Here's how the part is built. I have some questions about the finished solid (model axes, mm). Face numbers are marked on the shaded views. A direction names the side the tool comes from. Coordinates: 2 decimals unless noted, no trailing zeros. Loops run counter-clockwise (first coordinate to the right, second up) from the corner with the lowest first, then second, coordinate; pieces in that order, holes last. Notation, with made-up numbers: M 49,53.25 L 62,53.25 A33 cw 62,86.25 Z; hole C 76.25,-1 d3. An arc over 180 degrees is marked long. Use CSV: the item, a comma, the result in double quotes. Start each with the question number.
Q1. If we section it at C-C (z = -30): Please give me the cut outline in (x, y), and give its area (3 significant figures).
Q2. If we section it at A-A (x = 15): Please give me the cut outline in (y, z), and give its area (3 significant figures).
Q3. For pin 1 Ø2.5 at (x, z) = (9, -43.5) entering from -Y; pin 2 Ø1.5 at (x, z) = (11, -41.5) entering from +Y; pin 3 Ø8 at (x, y) = (7.5, 5) entering from -Z, each with a flat end and sliding along its axis, tell me the tip position at first contact or that it passes through.
Q4. Which directions (+Z, -Z, +X, -X, +Y, -Y) give clear straight access to the entire face, cutting with the end or side of a thin tool? Please do the marked faces 1, 2, 3 and 4.
Q5. If we section it at D-D (x = 10): Please give me the cut outline in (y, z), and give its area (3 significant figures).
Q6. Please list where these lines run through material, in increasing order: probe 1 along X at (y, z) = (28.55, 4.75); probe 2 along X at (y, z) = (28, 4); probe 3 along Z at (x, y) = (5.25, 11.5). Write a range as [from, to].
Q7. If we section it at B-B (y = 22): Please give me the cut outline in (x, z), and give its area (3 significant figures).
Q8. If we mould it in two halves opening along Y, with no side actions, what happens to the marked faces 5, 6 and 7? For each: +Y half, -Y half, draft (parallel to the pull), parting line (faces both ways), or undercut.
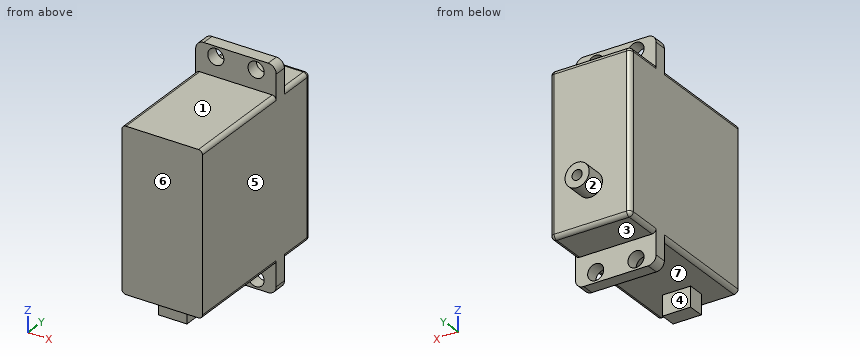
Autodesk Inventor part; units mm, degrees
ref_plane "作業平面1" through (0, 27.8, 0) normal (0, -1, 0) x (1, 0, 0)
ref_plane "作業平面2" through (0, 40.5, -20) normal (0, 0, 1) x (1, 0, 0)
ref_plane "作業平面3" through (0, 8, 0) normal (0, -1, 0) x (1, 0, 0)
sketch "スケッチ1" plane through (0, 0, 0) normal (0, 1, 0) x (-1, 0, 0)
  line L0 (0, 0) -> (-20, 0)
  line L1 (-20, 0) -> (-20, -40)
  line L2 (-20, -40) -> (0, -40)
  line L3 (0, -40) -> (0, 0)
  line L4 (0, -44.75) -> (-20, -44.75)
  line L5 (-20, -44.75) -> (-20, 4.75)
  line L6 (-20, 4.75) -> (0, 4.75)
  line L7 (0, 4.75) -> (0, -44.75)
  line L8 (-2, -47.25) -> (-18, -47.25)
  line L9 (-20, -45.25) -> (-20, 5.25)
  line L10 (-18, 7.25) -> (-2, 7.25)
  line L11 (0, 5.25) -> (0, -45.25)
  line L12 (-10, -61.4419) -> (-10, 22.3426)
  arc A0 (0, 5.25) -> (-2, 7.25) centre (-2, 5.25) ccw
  arc A1 (-18, 7.25) -> (-20, 5.25) centre (-18, 5.25) ccw
  arc A2 (-20, -45.25) -> (-18, -47.25) centre (-18, -45.25) ccw
  arc A3 (-2, -47.25) -> (0, -45.25) centre (-2, -45.25) ccw
  circle A4 centre (-10, -30) radius 3
  line L13 (-6.5, -45) -> (-13.5, -45)
  line L14 (-13.5, -45) -> (-13.5, -40)
  line L15 (-13.5, -40) -> (-6.5, -40)
  line L16 (-6.5, -40) -> (-6.5, -45)
  circle A5 centre (-10, -30) radius 1.25
  point P0 (-10, -20)
  point P1 (-20, 7.25)
  point P2 (-20, -47.25)
  point P3 (0, 7.25)
  point P4 (-5, 4.75)
  point P5 (-15, 4.75)
  point P6 (-20, 4.75)
  point P7 (-6.5, 0)
  point P8 (-13.5, 0)
  dimension "d0" = 20
  dimension "d1" = 40
  dimension "d2" = 20
  dimension "d3" = 49.5
  dimension "d4" = 20
  dimension "d5" = 54.5
  dimension "d6" = 24.75
  dimension "d7" = 27.25
  dimension "d8" = 10
  dimension "d9" = 0
  dimension "d10" = 0
  dimension "d11" = 4.75
  dimension "d12" = 0
  dimension "d13" = 10
  dimension "d14" = 10
  dimension "d15" = 5
  dimension "d16" = 2
  dimension "d30" = 6
  dimension "d33" = 7
  dimension "d34" = 5
  dimension "d35" = 3.5
  dimension "d42" = 2.5
  dimension "d45" = 0
extrude "押し出し1" add sketch "スケッチ1" along normal blind 40.5 contours L3 L2 L12 A4 L0 | L12 A4 L2 L1 L0 | A4 L12 A5 | L12 A5 A4 | A5 L12 | L12 A5
ref_plane "作業平面1" through (0, 27.8, 0) normal (0, -1, 0) x (1, 0, 0)
extrude "押し出し2" add sketch "スケッチ1" along normal blind 3.1 from surface at 27.8 contours L0 L12 L6 L7 | L0 L5 L6 L12 | L7 L4 L16 L2 | L6 L12 L10 A0 L11 | L6 L9 A1 L10 L12 | L16 L4 L12 L2 | L11 A3 L8 L12 L13 L16 L4 | L2 L14 L4 L5 | L12 L4 L14 L2 | L16 L13 L12 L4 | L4 L14 L13 L12 L8 A2 L9 | L12 L13 L14 L4
hole "穴1" at (5, 0, 4.75) at (15, 0, 4.75) direction (0, 1, 0) diameter 4 end through all
ref_plane "作業平面2" through (0, 40.5, -20) normal (0, 0, 1) x (1, 0, 0)
mirror "ミラー1" about plane through (0, 40.5, -20) normal (0, 0, 1) of "穴1"
extrude "押し出し3" add sketch "スケッチ1" along normal blind 5 from surface at 40.5 contours A4 L12 A5 | L12 A5 A4 | A5 L12 | L12 A5
ref_plane "作業平面3" through (0, 8, 0) normal (0, -1, 0) x (1, 0, 0)
extrude "押し出し4" add sketch "スケッチ1" against normal blind 4 from surface at 8 contours L16 L4 L12 L2 | L12 L4 L14 L2 | L16 L13 L12 L4 | L12 L13 L14 L4
fillet "フィレット1" radius 1 12 edges at (0, 35.7, 0) (0, 13.9, 0) (20, 13.9, 0) (20, 35.7, 0) (20, 13.9, -40) (20, 35.7, -40) (0, 13.9, -40) (0, 35.7, -40) (20, 40.5, -20) (0, 40.5, -20) (10, 40.5, 0) (10, 40.5, -40)
extrude "押し出し5" cut sketch "スケッチ1" against normal blind 4 from surface at 45.5 contours A5 L12 | L12 A5
equation "\"d35\" = 0.5 * d33"
properties part number "ServoMotor(20kg・cm)"
Results below:
1,outline,"M 0,0 L 20,0 L 20,39.5 A1 ccw 19,40.5 L 13,40.5 L 13,45.5 L 11.25,45.5 L 11.25,41.5 L 8.75,41.5 L 8.75,45.5 L 7,45.5 L 7,40.5 L 1,40.5 A1 ccw 0,39.5 Z"
1,area,"830 mm^2"
2,outline,"M 0,-40 L 27.8,-40 L 27.8,-42.75 L 30.9,-42.75 L 30.9,-40 L 39.5,-40 A1 ccw 40.5,-39 L 40.5,-1 A1 ccw 39.5,0 L 30.9,0 L 30.9,2.75 L 27.8,2.75 L 27.8,0 L 0,0 Z; M 27.8,-47.25 L 30.9,-47.25 L 30.9,-46.75 L 27.8,-46.75 Z; M 27.8,6.75 L 30.9,6.75 L 30.9,7.25 L 27.8,7.25 Z"
2,area,"1,640 mm^2"
3,pin 1,"y = 4"
3,pin 2,"y = 30.9"
3,pin 3,"z = -45"
4,face 1,"+Z, +X, -X, -Y"
4,face 2,"+Y"
4,face 3,"-Z, +X, -X, +Y"
4,face 4,"-Z, +X, -X"
5,outline,"M 0,-40 L 4,-40 L 4,-45 L 8,-45 L 8,-40 L 27.8,-40 L 27.8,-47.25 L 30.9,-47.25 L 30.9,-40 L 39.5,-40 A1 ccw 40.5,-39 L 40.5,-33 L 45.5,-33 L 45.5,-31.25 L 41.5,-31.25 L 41.5,-28.75 L 45.5,-28.75 L 45.5,-27 L 40.5,-27 L 40.5,-1 A1 ccw 39.5,0 L 30.9,0 L 30.9,7.25 L 27.8,7.25 L 27.8,0 L 0,0 Z"
5,area,"1,700 mm^2"
6,probe 1,"[0, 3], [7, 13], [17, 20]"
6,probe 2,"[0, 3.15], [6.85, 13.15], [16.85, 20]"
6,probe 3,"[-40, 0]"
7,outline,"M 0,-39 A1 ccw 1,-40 L 19,-40 A1 ccw 20,-39 L 20,-1 A1 ccw 19,0 L 1,0 A1 ccw 0,-1 Z"
7,area,"799 mm^2"
8,face 5,"draft"
8,face 6,"-Y half"
8,face 7,"undercut"
